from build123d import *

# Parameters (mm, degrees)
SKETCH_2_W           = 24
SKETCH_2_H           = 8
EXTRUDE_1_DEPTH      = 1
EXTRUDE_3_DEPTH      = 3
EXTRUDE_3_DEPTH_BACK = 3
EXTRUDE_5_REACH      = 45.174
SKETCH_7_W           = 24
SKETCH_7_H           = 4.701778719
SKETCH_3_R           = 1.5
CUT_EXTRUDE_1_DEPTH  = 43.614551505
FILLET_1_R           = 3


with BuildPart() as part:
    # Sketch 2 → Extrude 1 (new body)
    with BuildSketch(Plane(origin=(0, 0, 0), x_dir=(1, 0, 0), z_dir=(0, 1, 0))):
        Rectangle(SKETCH_2_W, SKETCH_2_H)
    extrude(amount=-EXTRUDE_1_DEPTH)

    # Extrude 5: up to this face of the body (flat: up to its plane)
    extrude_5_end = Plane(part.part.faces().sort_by_distance((0, -0.5, -4))[0])
    # Sketch 7 → Extrude 5 (add, up to the picked face)
    with BuildSketch(Plane.XY.offset(4), mode=Mode.PRIVATE) as extrude_5_sk1:
        with Locations((0, -2.350889359)):
            Rectangle(SKETCH_7_W, SKETCH_7_H)
    extrude_5_tool1 = split(extrude(extrude_5_sk1.sketch, amount=-EXTRUDE_5_REACH, mode=Mode.PRIVATE), bisect_by=extrude_5_end, keep=Keep.BOTH, mode=Mode.PRIVATE)


with BuildPart() as body_2:
    # Sketch 5 → Extrude 3 (new, two sides: drawn at the far end of the back side and taken through both)
    with BuildSketch(Plane.XY.offset(-EXTRUDE_3_DEPTH_BACK)):
        with BuildLine():
            ThreePointArc((30, -30), (21.213203436, -8.786796564), (0, 0))
            Line((0, 0), (0, -2))
            ThreePointArc((0, -2), (19.798989873, -10.201010127), (28, -30))
            Line((28, -30), (30, -30))
        make_face()
        with BuildLine():
            Line((0, -2), (0, 0))
            ThreePointArc((0, 0), (-21.213203436, -8.786796564), (-30, -30))
            Line((-30, -30), (-28, -30))
            ThreePointArc((-28, -30), (-19.798989873, -10.201010127), (0, -2))
        make_face()
    extrude(amount=EXTRUDE_3_DEPTH + EXTRUDE_3_DEPTH_BACK)


with BuildPart() as part_1:
    add(part.part)

    add(body_2.part)  # Extrude 5 merges body 2
    add(extrude_5_tool1.solids().sort_by(Axis((0, -2.350889, 4), (0, 0, -1)))[0])

    # Sketch 3 → Cut-Extrude 1 (cut, through all)
    with BuildSketch(Plane(origin=(0, 0, 0), x_dir=(1, 0, 0), z_dir=(0, 1, 0))):
        with Locations(Location((-7, 0, 0), (0, 0, 270))):
            Circle(SKETCH_3_R)
        with Locations(Location((7, 0, 0), (0, 0, 270))):
            Circle(SKETCH_3_R)
    extrude(amount=-CUT_EXTRUDE_1_DEPTH, mode=Mode.SUBTRACT)

    # Fillet 1
    # the kernel refuses this fillet: 3 mm, written as the material it takes off along each edge
    with BuildSketch(Plane(origin=(-12, -12.201778719, 4), x_dir=(0, 0, -1), z_dir=(0, 1, 0))) as fillet_1_piece_1_section:
        with BuildLine():
            CenterArc((FILLET_1_R, -FILLET_1_R), FILLET_1_R, 90, 90)
            Line((0, -FILLET_1_R), (0, 0))
            Line((0, 0), (FILLET_1_R, 0))
        make_face()
    fillet_1_piece_1 = extrude(amount=19.701778719, mode=Mode.PRIVATE)
    fillet_1_piece_1 = split(fillet_1_piece_1, bisect_by=Plane(origin=(-10.804220272, -4.438855897, 3), z_dir=(0, 0, 1)), keep=Keep.TOP, mode=Mode.PRIVATE)
    add(fillet_1_piece_1, mode=Mode.SUBTRACT)
    with BuildSketch(Plane(origin=(-12, -12.201778719, 4), x_dir=(0, 0, -1), z_dir=(0, 1, 0))) as fillet_1_piece_2_section:
        with BuildLine():
            CenterArc((FILLET_1_R, -FILLET_1_R), FILLET_1_R, 90, 90)
            Line((0, -FILLET_1_R), (0, 0))
            Line((0, 0), (FILLET_1_R, 0))
        make_face()
    fillet_1_piece_2 = extrude(amount=19.701778719, mode=Mode.PRIVATE)
    fillet_1_piece_2 = fillet_1_piece_2 - Plane(origin=(0, -30, 2.5069518), x_dir=(1, 0, 0), z_dir=(0, 0, -1)) * Cylinder(30, 52, mode=Mode.PRIVATE)
    add(fillet_1_piece_2, mode=Mode.SUBTRACT)
    with BuildSketch(Plane(origin=(-12, -12.201778719, -4), x_dir=(1, 0, 0), z_dir=(0, 1, 0))) as fillet_1_piece_3_section:
        with BuildLine():
            CenterArc((FILLET_1_R, -FILLET_1_R), FILLET_1_R, 90, 90)
            Line((0, -FILLET_1_R), (0, 0))
            Line((0, 0), (FILLET_1_R, 0))
        make_face()
    fillet_1_piece_3 = extrude(amount=19.701778719, mode=Mode.PRIVATE)
    fillet_1_piece_3 = split(fillet_1_piece_3, bisect_by=Plane(origin=(-10.804220065, -4.438855826, -3), z_dir=(0, 0, -1)), keep=Keep.TOP, mode=Mode.PRIVATE)
    add(fillet_1_piece_3, mode=Mode.SUBTRACT)
    with BuildSketch(Plane(origin=(-12, -12.201778719, -4), x_dir=(1, 0, 0), z_dir=(0, 1, 0))) as fillet_1_piece_4_section:
        with BuildLine():
            CenterArc((FILLET_1_R, -FILLET_1_R), FILLET_1_R, 90, 90)
            Line((0, -FILLET_1_R), (0, 0))
            Line((0, 0), (FILLET_1_R, 0))
        make_face()
    fillet_1_piece_4 = extrude(amount=19.701778719, mode=Mode.PRIVATE)
    fillet_1_piece_4 = fillet_1_piece_4 - Plane(origin=(0, -30, -2.506951801), x_dir=(1, 0, 0), z_dir=(0, 0, -1)) * Cylinder(30, 52, mode=Mode.PRIVATE)
    add(fillet_1_piece_4, mode=Mode.SUBTRACT)
    with BuildSketch(Plane(origin=(12, 7.5, 4), x_dir=(0, 0, -1), z_dir=(0, -1, 0))) as fillet_1_piece_5_section:
        with BuildLine():
            CenterArc((FILLET_1_R, -FILLET_1_R), FILLET_1_R, 90, 90)
            Line((0, -FILLET_1_R), (0, 0))
            Line((0, 0), (FILLET_1_R, 0))
        make_face()
    fillet_1_piece_5 = extrude(amount=19.701778719, mode=Mode.PRIVATE)
    fillet_1_piece_5 = fillet_1_piece_5 - Plane(origin=(0, -30, 2.506951802), x_dir=(1, 0, 0), z_dir=(0, 0, -1)) * Cylinder(30, 52, mode=Mode.PRIVATE)
    add(fillet_1_piece_5, mode=Mode.SUBTRACT)
    with BuildSketch(Plane(origin=(12, 7.5, 4), x_dir=(0, 0, -1), z_dir=(0, -1, 0))) as fillet_1_piece_6_section:
        with BuildLine():
            CenterArc((FILLET_1_R, -FILLET_1_R), FILLET_1_R, 90, 90)
            Line((0, -FILLET_1_R), (0, 0))
            Line((0, 0), (FILLET_1_R, 0))
        make_face()
    fillet_1_piece_6 = extrude(amount=19.701778719, mode=Mode.PRIVATE)
    fillet_1_piece_6 = split(fillet_1_piece_6, bisect_by=Plane(origin=(11.186935792, -3.254885209, 3), z_dir=(0, 0, 1)), keep=Keep.TOP, mode=Mode.PRIVATE)
    add(fillet_1_piece_6, mode=Mode.SUBTRACT)
    with BuildSketch(Plane(origin=(12, 7.5, -4), x_dir=(-1, 0, 0), z_dir=(0, -1, 0))) as fillet_1_piece_7_section:
        with BuildLine():
            CenterArc((FILLET_1_R, -FILLET_1_R), FILLET_1_R, 90, 90)
            Line((0, -FILLET_1_R), (0, 0))
            Line((0, 0), (FILLET_1_R, 0))
        make_face()
    fillet_1_piece_7 = extrude(amount=19.701778719, mode=Mode.PRIVATE)
    fillet_1_piece_7 = split(fillet_1_piece_7, bisect_by=Plane(origin=(11.240609722, -1.095811506, -3), z_dir=(0, 0, -1)), keep=Keep.TOP, mode=Mode.PRIVATE)
    add(fillet_1_piece_7, mode=Mode.SUBTRACT)
    with BuildSketch(Plane(origin=(12, 7.5, -4), x_dir=(-1, 0, 0), z_dir=(0, -1, 0))) as fillet_1_piece_8_section:
        with BuildLine():
            CenterArc((FILLET_1_R, -FILLET_1_R), FILLET_1_R, 90, 90)
            Line((0, -FILLET_1_R), (0, 0))
            Line((0, 0), (FILLET_1_R, 0))
        make_face()
    fillet_1_piece_8 = extrude(amount=19.701778719, mode=Mode.PRIVATE)
    fillet_1_piece_8 = fillet_1_piece_8 - Plane(origin=(0, -30, -2.506951802), x_dir=(1, 0, 0), z_dir=(0, 0, -1)) * Cylinder(30, 52, mode=Mode.PRIVATE)
    add(fillet_1_piece_8, mode=Mode.SUBTRACT)


solid = part_1.part
Verification items for the finished model (mm, model axes). A direction names the side the tool comes from. Round coordinates to 2 decimals unless told otherwise and drop trailing zeros. Loops run counter-clockwise (first coordinate to the right, second up) from the corner with the lowest first, then second, coordinate; pieces in that order, holes last. Notation, with made-up numbers: (-3.75, 0) - (21.25, 0) arc R19 cw to (21.25, 21) - close; hole circle Ø1 at (14.25, 89). An arc over 180 degrees is marked (long way). Use a Markdown table: item, result. Add a question column.
1. Release check for a two-part mould opening along X. For faces 6 (the face through (0, -4.702, 0)), 7 (the face through (5.536, -2.318, -0.325)), 8 (the face through (-10.69, -1.86, -3.48)), 9 (the face through (0, -2, -4)) record: released by +X, released by -X, zero draft, split by the parting line, or undercut.
2. Section check B-B, the plane x = 7. Record the boundary of the cut face in (y, z), plus the area to 3 significant figures.
3. Access from +Z, -Z, +X, -X, +Y, -Y to the whole of each face (thin tool, end or side, straight path). Record for faces 1 (the face through (24, -15, -3)), 2 (the face through (-23.4, -14, -3)), 3 (the face through (-24, -15, 3)), 4 (the face through (-10.748, -1.861, 3.438)), 5 (the face through (12, -1, 0)).
4. Gauge pin test, flat ends, axial feed: pin 1 (2 mm diameter, centred on x = 15.5, z = 2.5, fed in from -Y); pin 2 (2.5 mm diameter, centred on x = 5, z = -1.5, fed in from -Y); pin 3 (3 mm diameter, centred on y = -12, z = -2.5, fed in from +X); pin 4 (6 mm diameter, centred on x = 10, y = -4, fed in from +Z). Record the tip position at first contact, or that the pin passes through.
5. Section check D-D, the plane x = -2. Record the boundary of the cut face in (y, z), plus the area to 3 significant figures.
6. Section check C-C, the plane y = -22. Record the boundary of the cut face in (x, z).
7. Thickness scan on probe 1 along X at (y, z) = (-1.15, 0); probe 2 along X at (y, z) = (-2.75, 0); probe 3 along X at (y, z) = (-6, -0.5). Record the ranges inside material, lowest first. Write a range as [from, to].
8. Section check A-A, the plane z = 0. Record the boundary of the cut face in (x, y), plus the area to 3 significant figures.
Checks:
| question | item | result |
|---|---|---|
| 1 | face 6 | undercut |
| 1 | face 7 | undercut |
| 1 | face 8 | released by -X |
| 1 | face 9 | zero draft |
| 2 | outline | (-4.7, -4) - (0, -4) - (0, -1.5) - (-4.7, -1.5) - close; (-4.7, 1.5) - (0, 1.5) - (0, 4) - (-4.7, 4) - close |
| 2 | area | 23.5 mm^2 |
| 3 | face 1 | -Z, +X, +Y, -Y |
| 3 | face 2 | -Z, -X, +Y, -Y |
| 3 | face 3 | +Z, -X, +Y, -Y |
| 3 | face 4 | +Z, -X, +Y |
| 3 | face 5 | +Z, -Z, +X, +Y |
| 4 | pin 1 | stops at y = -7.38 |
| 4 | pin 2 | stops at y = -4.7 |
| 4 | pin 3 | stops at x = 25.05 |
| 4 | pin 4 | stops at z = 4 |
| 5 | outline | (-4.7, -4) - (0, -4) - (0, 4) - (-4.7, 4) - close |
| 5 | area | 37.6 mm^2 |
| 6 | outline | (-28.91, -3) - (-26.83, -3) - (-26.83, 3) - (-28.91, 3) - close; (26.83, -3) - (28.91, -3) - (28.91, 3) - (26.83, 3) - close |
| 7 | probe 1 | x = [-12, -8.5], [-5.5, 5.5], [8.5, 12] |
| 7 | probe 2 | x = [-12.55, -8.5], [-5.5, 5.5], [8.5, 12.55] |
| 7 | probe 3 | x = [-18, -14.42], [14.42, 18] |
| 8 | outline | (-30, -30) - (-28, -30) arc R28 cw to (-12, -4.7) - (-8.5, -4.7) - (-8.5, 0) - (-12, 0) - (-12, -2.5) arc R30 ccw to start; (-5.5, -4.7) - (5.5, -4.7) - (5.5, 0) - (-5.5, 0) - close; (8.5, -4.7) - (12, -4.7) arc R28 cw to (28, -30) - (30, -30) arc R30 ccw to (12, -2.5) - (12, 0) - (8.5, 0) - close |
| 8 | area | 217 mm^2 |
